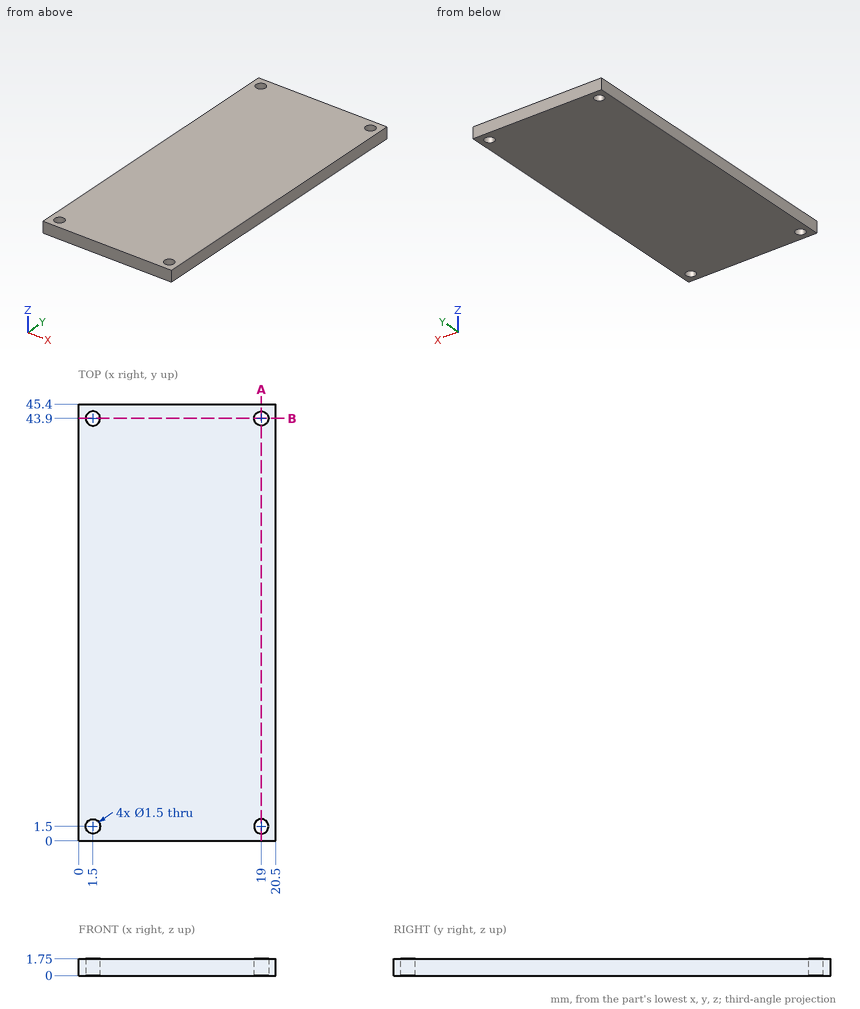
Could you check a few things on this drawing? It's one solid part, dimensions in mm from its lowest x, y, z. Round coordinates to 2 decimals unless told otherwise and drop trailing zeros. Order: outer loops, then holes, each group sorted by start corner. A loop starts at its lowest first (then second) coordinate and runs counter-clockwise, first axis right, second up.
(1) I'm going to push a flat-ended pin straight in: pin 1 (1.2 mm diameter, centred on x = 1.5, y = 1.5, fed in from -Z). Where does the tip first touch, or does it pass through?
Response values:
pin 1: passes through
(2) Please list where these lines run through material, in increasing order: line 1 along Y through (x, z) = (1.5, 0.8); line 2 along X through (y, z) = (43.9, 1.25); line 3 along X through (y, z) = (2, 1.65).
Response values:
line 1: y = 0 to 0.75, 2.25 to 43.15, 44.65 to 45.4
line 2: x = 0 to 0.75, 2.25 to 18.25, 19.75 to 20.5
line 3: x = 0 to 0.94, 2.06 to 18.44, 19.56 to 20.5
(3) Imagine slicing it at A-A (x = 19). Write out the boundary of the cut face in (y, z), plus the area to 3 significant figures.
Response values:
outline: (0, 0) - (0.75, 0) - (0.75, 1.75) - (0, 1.75) - close; (2.25, 0) - (43.15, 0) - (43.15, 1.75) - (2.25, 1.75) - close; (44.65, 0) - (45.4, 0) - (45.4, 1.75) - (44.65, 1.75) - close
area: 74.2 mm2
(4) Imagine slicing it at B-B (y = 43.9). Write out the boundary of the cut face in (x, z), plus the area to 3 significant figures.
Response values:
outline: (0, 0) - (0.75, 0) - (0.75, 1.75) - (0, 1.75) - close; (2.25, 0) - (18.25, 0) - (18.25, 1.75) - (2.25, 1.75) - close; (19.75, 0) - (20.5, 0) - (20.5, 1.75) - (19.75, 1.75) - close
area: 30.6 mm2
